Part print with two shaded views. Sizes in mm from the minimum x, y, z corner. Coordinates: 2 decimals unless noted, no trailing zeros. Loops run counter-clockwise (first coordinate to the right, second up) from the corner with the lowest first, then second, coordinate; pieces in that order, holes last.
Item 1: Flat gauge pins, fed straight in: pin 1 (3.5 mm diameter, centred on x = 98, z = 2, fed in from -Y); pin 2 (3 mm diameter, centred on x = 94.5, y = 13, fed in from -Z). Where does each tip first touch, or does it go through?
Item 2: Cut at B-B (y = 130.5). List the corners of the cut face in (x, z), and give its area (3 significant figures).
Item 3: Drill centre lines: line 1 along Y through (x, z) = (94.5, 3.5); line 2 along X through (y, z) = (144, 2.25); line 3 along Y through (x, z) = (107, 6.75). Where is each one in solid material? Low to high.
Item 4: Cut at A-A (z = 5.25). List the corners of the cut face in (x, y), and give its area (3 significant figures).
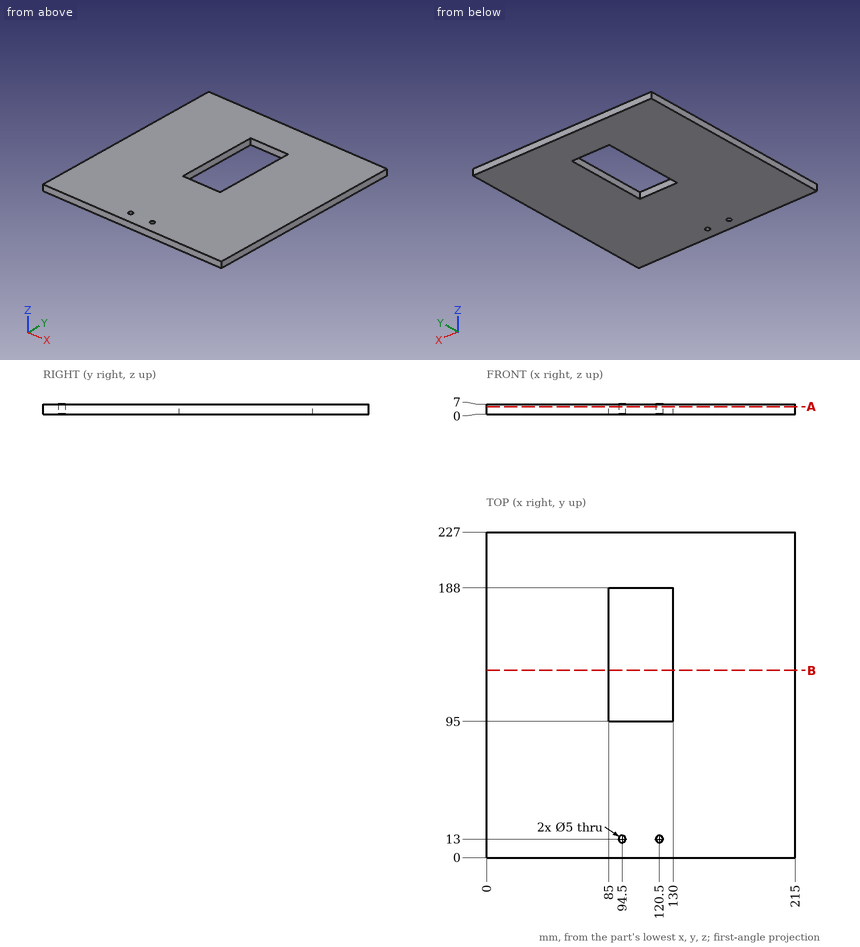
Filled sheet:
1. pin 1: stops at y = 0
1. pin 2: passes through
2. outline: (0, 0) - (85, 0) - (85, 7) - (0, 7) - close; (130, 0) - (215, 0) - (215, 7) - (130, 7) - close
2. area: 1,190 mm2
3. line 1: y = 0 to 10.5, 15.5 to 95, 188 to 227
3. line 2: x = 0 to 85, 130 to 215
3. line 3: y = 0 to 95, 188 to 227
4. outline: (0, 0) - (215, 0) - (215, 227) - (0, 227) - close; hole (85, 95) - (130, 95) - (130, 188) - (85, 188) - close; hole circle Ø5 at (94.5, 13); hole circle Ø5 at (120.5, 13)
4. area: 44,600 mm2
